```python
from build123d import *

# Parameters (mm, degrees)
RESSALTO_EXTRUS_O1_START         = 0.25
ESBO_O2_W                        = 30.5
ESBO_O2_H                        = 24.5
RESSALTO_EXTRUS_O1_DEPTH         = 3
ESBO_O3_W                        = 8.6
ESBO_O3_H                        = 24.5
RESSALTO_EXTRUS_O2_DEPTH         = 3
ESBO_O5_R                        = 4.25
CORTE_EXTRUS_O1_DEPTH            = 2
ESBO_O12_R                       = 3.25
CORTE_EXTRUS_O3_DEPTH            = 41.141904539
CBORE_FOR_M2_5_SHCS1_D           = 2.9
CBORE_FOR_M2_5_SHCS1_DEPTH       = 3
CBORE_FOR_M2_5_SHCS1_CBORE_D     = 5.5
CBORE_FOR_M2_5_SHCS1_CBORE_DEPTH = 2


with BuildPart() as part:
    # Esboço2 → Ressalto-extrusão1 (new body)
    with BuildSketch(Plane.XY.offset(RESSALTO_EXTRUS_O1_START)):
        with Locations((15, -9.25)):
            Rectangle(ESBO_O2_W, ESBO_O2_H)
    extrude(amount=RESSALTO_EXTRUS_O1_DEPTH)

    # Esboço3 → Ressalto-extrusão2 (add)
    with BuildSketch(Plane.ZY.offset(0.25)):
        with Locations((-1.05, -9.25)):
            Rectangle(ESBO_O3_W, ESBO_O3_H)
    ressalto_extrus_o2 = extrude(amount=RESSALTO_EXTRUS_O2_DEPTH)

    # Espelhar1: Ressalto-extrusão2 across plane
    add(ressalto_extrus_o2.mirror(Plane.ZY.offset(-15)))

    # Esboço5 → Corte-extrusão1 (cut)
    with BuildSketch(Plane.XY.offset(3.25)):
        with Locations((15, -6)):
            Circle(ESBO_O5_R)
    extrude(amount=-CORTE_EXTRUS_O1_DEPTH, mode=Mode.SUBTRACT)

    # Esboço12 → Corte-extrusão3 (cut, through all)
    with BuildSketch(Plane.XY.offset(1.25)):
        with Locations((15, -6)):
            Circle(ESBO_O12_R)
    extrude(amount=-CORTE_EXTRUS_O3_DEPTH, mode=Mode.SUBTRACT)

    # CBORE for M2.5 SHCS1
    with Locations(Plane.ZY.offset(3.25)):
        with Locations((-2.8, -1.5), (-2.8, -18.5)):
            cbore_for_m2_5_shcs1 = CounterBoreHole(CBORE_FOR_M2_5_SHCS1_D / 2, CBORE_FOR_M2_5_SHCS1_CBORE_D / 2, CBORE_FOR_M2_5_SHCS1_CBORE_DEPTH, depth=CBORE_FOR_M2_5_SHCS1_DEPTH)

    # Mirror1: CBORE for M2.5 SHCS1 across plane
    add(cbore_for_m2_5_shcs1.mirror(Plane.ZY.offset(-15)), mode=Mode.SUBTRACT)


solid = part.part
```
Read the model definition and answer for the solid it produces. Units are mm, in the model's axes. A direction names the side the tool comes from. Coordinates: 2 decimals unless noted, no trailing zeros. Loops run counter-clockwise (first coordinate to the right, second up) from the corner with the lowest first, then second, coordinate; pieces in that order, holes last.
(1) The part is cut by section A-A (x = 15). Determine the outline of the cut face in (y, z).
Solution:
outline: (-21.5, 0.25) - (-9.25, 0.25) - (-9.25, 1.25) - (-10.25, 1.25) - (-10.25, 3.25) - (-21.5, 3.25) - close; (-2.75, 0.25) - (3, 0.25) - (3, 3.25) - (-1.75, 3.25) - (-1.75, 1.25) - (-2.75, 1.25) - close
(2) The part is cut by section C-C (y = -18). Determine the outline of the cut face in (x, z).
Solution:
outline: (-3.25, -0.1) - (-1.25, -0.1) - (-1.25, -1.44) - (-0.25, -1.44) - (-0.25, 0.25) - (30.25, 0.25) - (30.25, -1.44) - (31.25, -1.44) - (31.25, -0.1) - (33.25, -0.1) - (33.25, 3.25) - (-3.25, 3.25) - close; (-1.25, -5.35) - (-0.25, -5.35) - (-0.25, -4.16) - (-1.25, -4.16) - close; (30.25, -5.35) - (31.25, -5.35) - (31.25, -4.16) - (30.25, -4.16) - close
(3) The part is cut by section B-B (y = -6). Determine the outline of the cut face in (x, z).
Solution:
outline: (-3.25, -5.35) - (-0.25, -5.35) - (-0.25, 0.25) - (11.75, 0.25) - (11.75, 1.25) - (10.75, 1.25) - (10.75, 3.25) - (-3.25, 3.25) - close; (18.25, 0.25) - (30.25, 0.25) - (30.25, -5.35) - (33.25, -5.35) - (33.25, 3.25) - (19.25, 3.25) - (19.25, 1.25) - (18.25, 1.25) - close
(4) The mould has two halves that part along Y. Classify faces 1 (the face through (-0.743, -19.916, -2.486)), 2 (the face through (15, 3, 1)), 3 (the face through (32, -9, -5.35)): released by +Y, released by -Y, zero draft, split by the parting line, or undercut.
Solution:
face 1: undercut
face 2: released by +Y
face 3: zero draft
(5) A tool of negligible diameter and unlimited length cuts with its end or side. For faces 4 (the face through (32.264, -1.606, -0.052)), 5 (the face through (30.25, -9, -3)), 6 (the face through (33.25, -9, 0)), 7 (the face through (-1.25, -3, -4)), from which of +Z, -Z, +X, -X, +Y, -Y can it reach the whole face along a straight path? Write none if from no direction.
Solution:
face 4: +X
face 5: -Z, +Y, -Y
face 6: +Z, -Z, +X, +Y, -Y
face 7: -X
(6) Consider line 1 along Y through (x, z) = (30.95, -2.8); line 2 along X through (y, z) = (-6.25, 2.5); line 3 along X through (y, z) = (-9.75, -2). Determine where each line is inside the solid, lowest interval first.
Solution:
line 1: y = -21.5 to -19.95, -17.05 to -2.95, -0.05 to 3
line 2: x = -3.25 to 10.76, 19.24 to 33.25
line 3: x = -3.25 to -0.25, 30.25 to 33.25
(7) Flat-ended cylindrical pins translate along their axes: pin 1 Ø2.5 at (y, z) = (-2, -4) entering from +X; pin 2 Ø8 at (x, y) = (6.5, -18.5) entering from -Z; pin 3 Ø2.5 at (y, z) = (-18.5, -2.8) entering from +X; pin 4 Ø2.5 at (x, y) = (17, -7) entering from +Z. Find the tip coordinate at first contact, or state that the pin passes through.
Solution:
pin 1: stops at x = 31.25
pin 2: stops at z = 0.25
pin 3: passes through
pin 4: stops at z = 1.25
(8) The part is cut by section D-D (z = -2.8). Count the separate pieces of the cut face and the enclosed holes in it, and give its area (3 significant figures).
Solution:
separate pieces: 6
enclosed holes: 0
area: 91.4 mm2
